Autodesk Inventor part; units mm, degrees
ref_plane "YZ Plane" through (0, 0, 0) normal (1, 0, 0) x (0, 1, 0)
ref_plane "XZ Plane" through (0, 0, 0) normal (0, 1, 0) x (-1, 0, 0)
ref_plane "XY Plane" through (0, 0, 0) normal (0, 0, 1) x (1, 0, 0)
sketch "Sketch1" plane through (0, 0, 0) normal (0, 0, 1) x (1, 0, 0)
  line L0 (0, 0) -> (60.96, 0)
  line L1 (60.96, 0) -> (60.96, 2.794) construction
  line L2 (60.96, 101.6) -> (0, 101.6)
  line L3 (0, 101.6) -> (0, 2.794)
  line L4 (-5.08, 0) -> (5.08, 0)
  line L5 (5.08, 0) -> (5.08, 2.794)
  line L6 (5.08, 2.794) -> (-5.08, 2.794)
  line L7 (-5.08, 2.794) -> (-5.08, 0) construction
  line L8 (15.24, 0) -> (25.4, 0)
  line L9 (25.4, 0) -> (25.4, 2.794)
  line L10 (25.4, 2.794) -> (15.24, 2.794)
  line L11 (15.24, 2.794) -> (15.24, 0)
  line L12 (35.56, 0) -> (45.72, 0)
  line L13 (45.72, 0) -> (45.72, 2.794)
  line L14 (45.72, 2.794) -> (35.56, 2.794)
  line L15 (35.56, 2.794) -> (35.56, 0)
  line L16 (55.88, 0) -> (66.04, 0) construction
  line L17 (66.04, 0) -> (66.04, 2.794) construction
  line L18 (66.04, 2.794) -> (55.88, 2.794)
  line L19 (55.88, 2.794) -> (55.88, 0)
  line L20 (60.96, 2.794) -> (60.96, 101.6)
  line L21 (0, 2.794) -> (0, 0) construction
  line L22 (0, 2.794) -> (5.08, 2.794)
  line L23 (5.08, 0) -> (5.08, 2.794)
  line L24 (5.08, 0) -> (15.24, 0)
  line L25 (15.24, 0) -> (15.24, 2.794)
  line L26 (15.24, 2.794) -> (25.4, 2.794)
  line L27 (25.4, 2.794) -> (25.4, 0)
  line L28 (25.4, 0) -> (35.56, 0)
  line L29 (35.56, 0) -> (35.56, 2.794)
  line L30 (35.56, 2.794) -> (45.72, 2.794)
  line L31 (45.72, 2.794) -> (45.72, 0)
  line L32 (45.72, 0) -> (55.88, 0)
  line L33 (55.88, 0) -> (55.88, 2.794)
  line L34 (55.88, 2.794) -> (60.96, 2.794)
  dimension "d0" = 10.16
  dimension "d1" = 2.794
  dimension "d5" = 20.32
  dimension "d11" = 101.6
  dimension "d14" = 5.08
  dimension "d15" = 5.08
extrude "Extrusion2" add sketch "Sketch1" along normal blind 5.08 contours L5 L6 L3 L2 L20 L18 L19 L0 L13 L14 L15 L9 L10 L11
sketch "Sketch2" plane through (0, 0, 5.08) normal (0, 0, 1) x (1, 0, 0)
  line L0 (33.3926, 34.8025) -> (40.5768, 27.6183)
  line L1 (36.9847, 38.3946) -> (44.1689, 31.2104)
  line L2 (58.5374, 16.8419) -> (61.3536, 14.0257)
  line L3 (61.3536, 14.0257) -> (94.79, 106.8091)
  line L4 (94.79, 106.8091) -> (9.0512, 130.8761)
  line L5 (9.0512, 130.8761) -> (-6.9479, 112.9626)
  line L6 (-6.9479, 112.9626) -> (0, 75.3793)
  line L7 (0, 101.6) -> (0, 2.794)
  line L8 (0, 75.3793) -> (58.5374, 16.8419)
  line L9 (36.9847, 38.3946) -> (33.3926, 34.8025)
  line L10 (40.5768, 27.6183) -> (44.1689, 31.2104)
  point P0 (0, 0)
extrude "Extrusion3" cut sketch "Sketch2" against normal blind 5.08 contours L8 L6 L5 L4 L3 L2 L1
sketch "Sketch3" plane through (0, 0, 5.08) normal (0, 0, 1) x (1, 0, 0)
  line L0 (33.3926, 34.8025) -> (40.5768, 27.6183)
  line L1 (36.9847, 38.3946) -> (44.1689, 31.2104)
  line L2 (60.96, 14.4193) -> (0, 75.3793)
  line L3 (58.5374, 16.8419) -> (51.3531, 24.0262)
  line L4 (51.3531, 24.0262) -> (47.761, 20.434)
  line L5 (47.761, 20.434) -> (54.9452, 13.2498)
  line L6 (54.9452, 13.2498) -> (58.5374, 16.8419)
  line L7 (44.1689, 31.2104) -> (36.9847, 38.3946)
  line L8 (36.9847, 38.3946) -> (33.3926, 34.8025)
  line L9 (33.3926, 34.8025) -> (40.5768, 27.6183)
  line L10 (40.5768, 27.6183) -> (44.1689, 31.2104)
  line L11 (29.8005, 45.5788) -> (22.6163, 52.763)
  line L12 (22.6163, 52.763) -> (19.0242, 49.1709)
  line L13 (19.0242, 49.1709) -> (26.2084, 41.9867)
  line L14 (26.2084, 41.9867) -> (29.8005, 45.5788)
  line L15 (15.4321, 59.9472) -> (8.2479, 67.1314)
  line L16 (8.2479, 67.1314) -> (4.6558, 63.5393)
  line L17 (4.6558, 63.5393) -> (11.84, 56.3551)
  line L18 (11.84, 56.3551) -> (15.4321, 59.9472)
  line L19 (1.0637, 74.3156) -> (-6.1205, 81.4998)
  line L20 (-6.1205, 81.4998) -> (-9.7126, 77.9077)
  line L21 (-9.7126, 77.9077) -> (-2.5284, 70.7235)
  line L22 (-2.5284, 70.7235) -> (1.0637, 74.3156)
  line L23 (-13.3047, 88.684) -> (-20.4889, 95.8682)
  line L24 (-20.4889, 95.8682) -> (-24.081, 92.2761)
  line L25 (-24.081, 92.2761) -> (-16.8968, 85.0919)
  line L26 (-16.8968, 85.0919) -> (-13.3047, 88.684)
  line L27 (36.9847, 38.3946) -> (33.3926, 34.8025)
  line L28 (40.5768, 27.6183) -> (44.1689, 31.2104)
  point P0 (0, 0)
  point P1 (46.5916, 28.7877)
  point P2 (26.2084, 41.9867)
  point P3 (32.2232, 43.1561)
  point P4 (11.84, 56.3551)
  point P5 (17.8548, 57.5245)
  point P6 (-2.5284, 70.7235)
  point P7 (3.4864, 71.8929)
  point P8 (-16.8968, 85.0919)
  point P9 (-10.882, 86.2613)
  dimension "d24" = 20.32
  dimension "d20" = 5.08
extrude "Extrusion4" cut sketch "Sketch3" against normal blind 5.08 contours L8 L1 L10 L0 | L22 L21 L20 L19 L2 | L18 L17 L16 L2 | L14 L13 L12 L2 | L2 L6 L5 L4
sketch "Sketch4" plane through (0, 0, 5.08) normal (0, 0, 1) x (1, 0, 0)
  line L0 (4.6558, 63.5393) -> (8.2479, 67.1314)
  line L1 (8.2479, 67.1314) -> (1.0637, 74.3156)
  line L2 (1.0637, 74.3156) -> (0, 73.2519)
  line L3 (0, 73.2519) -> (0, 2.794) construction
  line L4 (0, 2.794) -> (5.08, 2.794)
  line L5 (5.08, 2.794) -> (5.08, 0)
  line L6 (5.08, 0) -> (15.24, 0)
  line L7 (15.24, 0) -> (15.24, 2.794)
  line L8 (15.24, 2.794) -> (25.4, 2.794)
  line L9 (25.4, 2.794) -> (25.4, 0)
  line L10 (25.4, 0) -> (35.56, 0)
  line L11 (35.56, 0) -> (35.56, 2.794)
  line L12 (35.56, 2.794) -> (45.72, 2.794)
  line L13 (45.72, 2.794) -> (45.72, 0)
  line L14 (45.72, 0) -> (55.88, 0)
  line L15 (55.88, 0) -> (55.88, 2.794)
  line L16 (55.88, 2.794) -> (60.96, 2.794)
  line L17 (60.96, 2.794) -> (60.96, 14.4193)
  line L18 (60.96, 14.4193) -> (58.5374, 16.8419)
  line L19 (58.5374, 16.8419) -> (54.9452, 13.2498)
  line L20 (54.9452, 13.2498) -> (47.761, 20.434)
  line L21 (47.761, 20.434) -> (51.3531, 24.0262)
  line L22 (51.3531, 24.0262) -> (44.1689, 31.2104)
  line L23 (44.1689, 31.2104) -> (40.5768, 27.6183)
  line L24 (40.5768, 27.6183) -> (33.3926, 34.8025)
  line L25 (33.3926, 34.8025) -> (36.9847, 38.3946)
  line L26 (36.9847, 38.3946) -> (29.8005, 45.5788)
  line L27 (29.8005, 45.5788) -> (26.2084, 41.9867)
  line L28 (26.2084, 41.9867) -> (19.0242, 49.1709)
  line L29 (19.0242, 49.1709) -> (22.6163, 52.763)
  line L30 (22.6163, 52.763) -> (15.4321, 59.9472)
  line L31 (15.4321, 59.9472) -> (11.84, 56.3551)
  line L32 (11.84, 56.3551) -> (4.6558, 63.5393)
  line L33 (4.6558, 63.5393) -> (0, 58.8835)
  line L34 (0, 73.2519) -> (0, 2.794) construction
  line L35 (4.6558, 63.5393) -> (8.2479, 67.1314)
  line L36 (8.2479, 67.1314) -> (3.9736, 83.8978)
  line L37 (3.9736, 83.8978) -> (-8.4485, 80.2357)
  line L38 (-8.4485, 80.2357) -> (0, 58.8835)
  line L39 (4.6558, 63.5393) -> (8.2479, 67.1314)
  line L40 (8.2479, 67.1314) -> (3.9736, 83.8978)
  line L41 (0, 58.8835) -> (8.2479, 67.1314)
  line L42 (0, 58.8835) -> (-8.4485, 80.2357)
  point P0 (0, 0)
extrude "Extrusion5" cut sketch "Sketch4" against normal blind 5.08
equation "\"d5\" = 2 * d0"
equation "\"d24\" = 2 * d21"
properties part number "SledSideSupport" material "Wood (Birch)"
CAD build for the part. Positions are in the model's coordinates, mm. A direction names the side the tool comes from. Coordinates: 2 decimals unless noted, no trailing zeros. Write each loop counter-clockwise with the first axis right and the second up, starting at its lowest first coordinate (ties: lowest second). Pieces come first, ordered by that corner, then holes. Notation, with made-up numbers: (11, -6.75) -> (23, -6.75) arc R30 cw to (23, 21.25) -> close; hole circle Ø2 at (70, -8.75). An arc over 180 degrees is marked (long way). Use CSV: the item, a comma, the result in double quotes. Start each with the question number.
Item 1: Band-saw the part on A-A, the plane x = 20. Write the cut outline in (y, z), plus the area to 3 significant figures.
Item 2: Band-saw the part on B-B, the plane y = 16. Write the cut outline in (x, z) (3 decimals).
Item 3: Drop flat-ended pins along their axis: P1, Ø2, axis at y = 1, z = 1.5, coming from the +X side; P2, Ø0.8, axis at y = 1, z = 2.5, coming from the -X side; P3, Ø2.5, axis at x = 59, z = 3.5, coming from the -Y side. Give the stop position or say it passes through.
Item 4: Tool access for faces 1 (the flat face through (35.56, 1, 3)), 2 (the flat face through (20.845, 50.992, 2.576)), 3 (the flat face through (42.35, 29.39, 2.58)), 4 (the flat face through (55.88, 1, 3)): list every direction of +Z, -Z, +X, -X, +Y, -Y with a clear straight run to the whole face (end or side of a thin tool).
Item 5: Two-plate mould, pull along Y, no slides. Class faces 5 (the flat face through (35.21, 36.62, 2.58)), 6 (the flat face through (2.36, 61.244, 2.576)), 7 (the flat face through (5.08, 1, 3)): +Y half, -Y half, draft (parallel to the pull), parting line (faces both ways), or undercut.
Item 6: Wall check: probe 1 along X at (y, z) = (45.5, 0.75); probe 2 along Y at (x, z) = (50.5, 2.25) (3 decimals); probe 3 along X at (y, z) = (15, 0.65) (3 decimals). Give the ranges that are in metal, low to high.
Item 7: Band-saw the part on D-D, the plane x = 7. Write the cut outline in (y, z).
Response values:
1,outline,"(2.79, 0) -> (48.2, 0) -> (48.2, 5.08) -> (2.79, 5.08) -> close; (50.15, 0) -> (55.38, 0) -> (55.38, 5.08) -> (50.15, 5.08) -> close"
1,area,"257 mm2"
2,outline,"(0, 0) -> (52.195, 0) -> (52.195, 5.08) -> (0, 5.08) -> close; (57.695, 0) -> (59.379, 0) -> (59.379, 5.08) -> (57.695, 5.08) -> close"
3,P1,"stops at x = 55.88"
3,P2,"stops at x = 5.08"
3,P3,"stops at y = 2.79"
4,face 1,"+Z, -Z, -Y"
4,face 2,"+Z, -Z, +X"
4,face 3,"+Z, -Z, +Y"
4,face 4,"+Z, -Z, +X, -Y"
5,face 5,"undercut"
5,face 6,"+Y half"
5,face 7,"draft"
6,probe 1,"x = 0 to 22.7, 29.72 to 29.88"
6,probe 2,"y = 0 to 17.695, 23.173 to 24.879"
6,probe 3,"x = 0 to 53.195, 56.695 to 60.379"
7,outline,"(0, 0) -> (61.2, 0) -> (61.2, 5.08) -> (0, 5.08) -> close"
